The listing builds one solid part. Answer for the finished solid, in the listing's coordinates (mm). A direction names the side the tool comes from. Give positions to 0.01 mm unless a question says otherwise; leave off trailing zeros. One line per item, written item: value. Start each with the question number.
Q1. The mould has two halves that part along X. Classify faces 3 (the flat face through (20, -52, 493)), 4 (the flat face through (12, 20, 493)), 5 (the flat face through (-20, 12, 493)), 6 (the flat face through (16.4, -20, 493)): +X half, -X half, draft (parallel to the pull), parting line (faces both ways), or undercut.
Q2. A flat-ended cylindrical pin translates along its axis: pin 1 (5 mm diameter, centred on x = 4, z = 158, fed in from +Y). Find the tip coordinate at first contact, or state that the pin passes through.
Q3. A cutting plane is placed at A-A, the plane z = 898. State how many separate pieces and enclosed holes the cut face has, and give its area (3 significant figures).
Q4. Consider L1, parallel to Y at x = -13.5, z = 660.5; L2, parallel to X at y = -27.5, z = 299; L3, parallel to Y at x = -11, z = 192. Determine where each line is inside the solid, lowest interval first.
Q5. For faces 1 (the flat face through (20, 12, 493)), 2 (the flat face through (-16.4, -20, 493)), determine the directions among +Z, -Z, +X, -X, +Y, -Y from which every point of the face is accessible in a straight line to the end or side of a thin tool.
from build123d import *

# Parameters (mm, degrees)
SKETCH_1_R      = 4.25
SKETCH_1_R_2    = 3.4
EXTRUDE_1_DEPTH = 1000


with BuildPart() as part:
    # Эскиз1 → Бобышка-Вытянуть1 (new body)
    with BuildSketch(Plane.XY):
        with BuildLine():
            Line((-20, 19.5), (-20, 7))
            Line((-20, 7), (-20, 4.2))
            Line((-20, 4.2), (-16.5, 4.2))
            Line((-16.5, 4.2), (-16.5, 7))
            Line((-16.5, 7), (-9, 7))
            Line((-9, 7), (-9, 5.541660401))
            ThreePointArc((-9, 5.541660401), (-5.3, 0), (-9, -5.541660401))
            Line((-9, -5.541660401), (-9, -7))
            Line((-9, -7), (-16.5, -7))
            Line((-16.5, -7), (-16.5, -4.2))
            Line((-16.5, -4.2), (-20, -4.2))
            Line((-20, -4.2), (-20, -7))
            Line((-20, -7), (-20, -33))
            Line((-20, -33), (-20, -35.8))
            Line((-20, -35.8), (-16.5, -35.8))
            Line((-16.5, -35.8), (-16.5, -33))
            Line((-16.5, -33), (-9, -33))
            Line((-9, -33), (-9, -34.458339599))
            ThreePointArc((-9, -34.458339599), (-5.3, -40), (-9, -45.541660401))
            Line((-9, -45.541660401), (-9, -47))
            Line((-9, -47), (-16.5, -47))
            Line((-16.5, -47), (-16.5, -44.2))
            Line((-16.5, -44.2), (-20, -44.2))
            Line((-20, -44.2), (-20, -47))
            Line((-20, -47), (-20, -59.5))
            ThreePointArc((-20, -59.5), (-19.853553391, -59.853553391), (-19.5, -60))
            Line((-19.5, -60), (-7, -60))
            Line((-7, -60), (-4.2, -60))
            Line((-4.2, -60), (-4.2, -56.5))
            Line((-4.2, -56.5), (-7, -56.5))
            Line((-7, -56.5), (-7, -49))
            Line((-7, -49), (-5.541660401, -49))
            ThreePointArc((-5.541660401, -49), (0, -45.3), (5.541660401, -49))
            Line((5.541660401, -49), (7, -49))
            Line((7, -49), (7, -56.5))
            Line((7, -56.5), (4.2, -56.5))
            Line((4.2, -56.5), (4.2, -60))
            Line((4.2, -60), (7, -60))
            Line((7, -60), (19.5, -60))
            ThreePointArc((19.5, -60), (19.853553391, -59.853553391), (20, -59.5))
            Line((20, -59.5), (20, -47))
            Line((20, -47), (20, -44.2))
            Line((20, -44.2), (16.5, -44.2))
            Line((16.5, -44.2), (16.5, -47))
            Line((16.5, -47), (9, -47))
            Line((9, -47), (9, -45.541660401))
            ThreePointArc((9, -45.541660401), (5.3, -40), (9, -34.458339599))
            Line((9, -34.458339599), (9, -33))
            Line((9, -33), (16.5, -33))
            Line((16.5, -33), (16.5, -35.8))
            Line((16.5, -35.8), (20, -35.8))
            Line((20, -35.8), (20, -33))
            Line((20, -33), (20, -7))
            Line((20, -7), (20, -4.2))
            Line((20, -4.2), (16.5, -4.2))
            Line((16.5, -4.2), (16.5, -7))
            Line((16.5, -7), (9, -7))
            Line((9, -7), (9, -5.541660401))
            ThreePointArc((9, -5.541660401), (5.3, 0), (9, 5.541660401))
            Line((9, 5.541660401), (9, 7))
            Line((9, 7), (16.5, 7))
            Line((16.5, 7), (16.5, 4.2))
            Line((16.5, 4.2), (20, 4.2))
            Line((20, 4.2), (20, 7))
            Line((20, 7), (20, 19.5))
            ThreePointArc((20, 19.5), (19.853553391, 19.853553391), (19.5, 20))
            Line((19.5, 20), (7, 20))
            Line((7, 20), (4.2, 20))
            Line((4.2, 20), (4.2, 16.5))
            Line((4.2, 16.5), (7, 16.5))
            Line((7, 16.5), (7, 9))
            Line((7, 9), (5.541660401, 9))
            ThreePointArc((5.541660401, 9), (0, 5.3), (-5.541660401, 9))
            Line((-5.541660401, 9), (-7, 9))
            Line((-7, 9), (-7, 16.5))
            Line((-7, 16.5), (-4.2, 16.5))
            Line((-4.2, 16.5), (-4.2, 20))
            Line((-4.2, 20), (-7, 20))
            Line((-7, 20), (-19.5, 20))
            ThreePointArc((-19.5, 20), (-19.853553391, 19.853553391), (-20, 19.5))
        make_face()
        with Locations((-13.5, -53.5)):
            Circle(SKETCH_1_R, mode=Mode.SUBTRACT)
        with Locations((13.5, -53.5)):
            Circle(SKETCH_1_R, mode=Mode.SUBTRACT)
        with Locations((0, -40)):
            Circle(SKETCH_1_R_2, mode=Mode.SUBTRACT)
        with Locations((-13.5, 13.5)):
            Circle(SKETCH_1_R, mode=Mode.SUBTRACT)
        with BuildLine():
            Line((16.4, -10.5), (16.4, -29.5))
            Line((16.4, -29.5), (6, -29.5))
            ThreePointArc((6, -29.5), (0, -35.5), (-6, -29.5))
            Line((-6, -29.5), (-16.4, -29.5))
            Line((-16.4, -29.5), (-16.4, -10.5))
            Line((-16.4, -10.5), (-6, -10.5))
            ThreePointArc((-6, -10.5), (0, -4.5), (6, -10.5))
            Line((6, -10.5), (16.4, -10.5))
        make_face(mode=Mode.SUBTRACT)
        Circle(SKETCH_1_R_2, mode=Mode.SUBTRACT)
        with Locations((13.5, 13.5)):
            Circle(SKETCH_1_R, mode=Mode.SUBTRACT)
    extrude(amount=EXTRUDE_1_DEPTH)


solid = part.part
Answer block:
1. face 3: +X half
1. face 4: draft
1. face 5: -X half
1. face 6: undercut
2. pin 1: y = 20
3. separate pieces: 1
3. enclosed holes: 7
3. area: 1,180 mm^2
4. L1: -60 to -57.75, -49.25 to -47, -33 to -29.5, -10.5 to -7, 7 to 9.25, 17.75 to 20
4. L2: -20 to -16.4, 16.4 to 20
4. L3: -60 to -56.94, -50.06 to -47, -33 to -29.5, -10.5 to -7, 7 to 10.06, 16.94 to 20
5. face 1: +Z, -Z, +X, +Y, -Y
5. face 2: +Z, -Z
